Can you work these out from the model? Positions are in its coordinate system, mm. Face numbers are marked on the shaded views. A direction names the side the tool comes from. Coordinates: 2 decimals unless noted, no trailing zeros. Order: outer loops, then holes, each group sorted by start corner. A loop starts at its lowest first (then second) coordinate and runs counter-clockwise, first axis right, second up. Notation, with made-up numbers: M 54.25,17.5 L 72.25,17.5 A19 ccw 72.25,54.5 Z; hole C 82,57.25 d10. An arc over 180 degrees is marked long. Answer as a JSON object with one key per item and string values.
from build123d import *

# Parameters (mm, degrees)
F0_R     = 16.201706
F1_DEPTH = 6
F2_R     = 2


with BuildPart() as f1:
    # F0 (on Top) → F1 (new body)
    with BuildSketch(Plane.XY):
        Circle(F0_R)
        Polygon((-12.701706, 0), (-6.350853, 11), (6.350853, 11), (12.701706, 0), (6.350853, -11), (-6.350853, -11), align=None, mode=Mode.SUBTRACT)
    extrude(amount=F1_DEPTH)

    # F2
    f2_edges = [f1.edges().sort_by_distance(p)[0] for p in [
        (-16.201706, 0, 6),
        (-16.201706, 0, 0),
    ]]
    fillet(f2_edges, radius=F2_R)


solid = f1.part
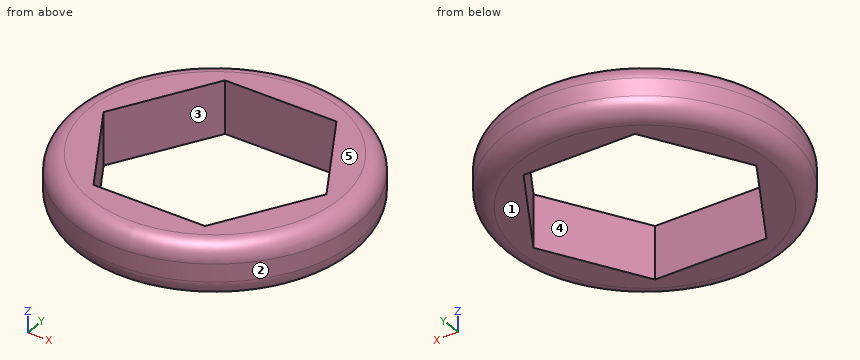
Item 1: I'm going to push flat-ended pins straight in: pin 1 (1 mm diameter, centred on x = -4, z = 4.5, fed in from +Y); pin 2 (3 mm diameter, centred on y = 11.5, z = 1, fed in from +X). Where does each tip first touch, or does it pass through?
Answers follow:
{"pin 1": "stops at y = 15.79", "pin 2": "stops at x = 12.6"}
Item 2: I want a section at A-A, the plane x = 0. Write out the boundary of the cut face in (y, z).
Answers follow:
{"outline": "M -16.2,2 A2 ccw -14.2,0 L -11,0 L -11,6 L -14.2,6 A2 ccw -16.2,4 Z; M 11,0 L 14.2,0 A2 ccw 16.2,2 L 16.2,4 A2 ccw 14.2,6 L 11,6 Z"}
Item 3: I want a section at B-B, the plane z = 5.25. Write out the boundary of the cut face in (x, y).
Answers follow:
{"outline": "C 0,0 d31.53; hole M -12.7,0 L -6.35,-11 L 6.35,-11 L 12.7,0 L 6.35,11 L -6.35,11 Z"}
Item 4: Which directions (+Z, -Z, +X, -X, +Y, -Y) give clear straight access to the entire face, cutting with the end or side of a thin tool? Please do the marked faces 4 and 5.
Answers follow:
{"face 4": "+Z, -Z", "face 5": "+Z, +X, -X, +Y, -Y"}
Item 5: If we mould it in two halves opening along Y, with no side actions, what happens to the marked faces 1, 2 and 3? For each: pulls with the +Y half, pulls with the -Y half, needs draft (parallel to the pull), parting line crosses it, or undercut.
Answers follow:
{"face 1": "needs draft", "face 2": "parting line crosses it", "face 3": "undercut"}
Item 6: Please list where these lines run through material, in increasing order: line 1 (Y direction, x = 3.5, z = 0.4); line 2 (X direction, y = -8.5, z = 4.85); line 3 (X direction, y = -6.5, z = 5).
Answers follow:
{"line 1": "y = -15 to -11, 11 to 15", "line 2": "x = -13.57 to -7.79, 7.79 to 13.57", "line 3": "x = -14.55 to -8.95, 8.95 to 14.55"}
